Design review of the part built by this model. Coordinates are the model's own, in mm. A direction names the side the tool comes from. Give positions to 0.01 mm unless a question says otherwise; leave off trailing zeros. Order: outer loops, then holes, each group sorted by start corner. A loop starts at its lowest first (then second) coordinate and runs counter-clockwise, first axis right, second up. Notation, with made-up numbers: (28, -10.75) -> (51, -10.75) arc R24 ccw to (51, 27.25) -> close; hole circle Ø3 at (-4.5, -20). An arc over 180 degrees is marked (long way). Return JSON: item names as keys, results as strings.
```python
from build123d import *

# Parameters (mm, degrees)
AUFSATZ_LINEAR_START            = -9.5
AUFSATZ_LINEAR_AUSTRAGEN1_DEPTH = 80


with BuildPart() as part:
    # Skizze1 → Aufsatz-Linear austragen1 (new body)
    with BuildSketch(Plane.XY.offset(AUFSATZ_LINEAR_START)):
        with BuildLine():
            Line((0, 25), (435, 25))
            Line((435, 25), (450, 25))
            ThreePointArc((450, 25), (475, 0), (450, -25))
            Line((450, -25), (0, -25))
            ThreePointArc((0, -25), (-25, 0), (0, 25))
        make_face()
        with BuildLine():
            Line((0, 23), (435, 23))
            Line((435, 23), (450, 23))
            ThreePointArc((450, 23), (473, 0), (450, -23))
            Line((450, -23), (0, -23))
            ThreePointArc((0, -23), (-23, 0), (0, 23))
        make_face(mode=Mode.SUBTRACT)
    extrude(amount=-AUFSATZ_LINEAR_AUSTRAGEN1_DEPTH)


solid = part.part
```
Item 1: Add section A-A (y = 0). Give the boundary of the cut face in (x, z).
Result set:
{"outline": "(-25, -89.5) -> (-23, -89.5) -> (-23, -9.5) -> (-25, -9.5) -> close; (473, -89.5) -> (475, -89.5) -> (475, -9.5) -> (473, -9.5) -> close"}
Item 2: Machinability: for faces 1 (the face through (226, -24, -9.5)), 2 (the face through (-22.994, -0.506, -48.94)), which of the approach directions +Z, -Z, +X, -X, +Y, -Y give a long, thin tool a straight path to every point of the face, cutting with its end or side? Answer none if there is none.
Result set:
{"face 1": "+Z, +X, -X, +Y, -Y", "face 2": "+Z, -Z"}
Item 3: Mouldability with a two-part tool opening along Y and no side actions: class faces 3 (the face through (228, -25, -49)), 4 (the face through (226, -24, -89.5)), 5 (the face through (228, -23, -49)) as released by +Y, released by -Y, zero draft, split by the parting line, or undercut.
Result set:
{"face 3": "released by -Y", "face 4": "zero draft", "face 5": "undercut"}
Item 4: Add section B-B (x = 57.5). Give the boundary of the cut face in (y, z), plus the area to 3 significant figures.
Result set:
{"outline": "(-25, -89.5) -> (-23, -89.5) -> (-23, -9.5) -> (-25, -9.5) -> close; (23, -89.5) -> (25, -89.5) -> (25, -9.5) -> (23, -9.5) -> close", "area": "320 mm^2"}
Item 5: For pin 1 (6 mm diameter, centred on y = 13.5, z = -65, fed in from -X); pin 2 (2 mm diameter, centred on y = 8, z = -29, fed in from -X); pin 3 (10 mm diameter, centred on x = 416, y = -15, fed in from +Z) (3 decimals); pin 4 (4 mm diameter, centred on y = 3, z = -32.5, fed in from -X), all flat-tipped, find the tip position at first contact; note any pin that passes through.
Result set:
{"pin 1": "stops at x = -22.69", "pin 2": "stops at x = -24", "pin 3": "passes through", "pin 4": "stops at x = -24.98"}
Item 6: Wall thickness on L1, parallel to Y at x = 254, z = -33.5; L2, parallel to X at y = -2, z = -24; L3, parallel to X at y = -10.5, z = -39: over which ranges is each line inside the solid? List them lowest first. Write a range as [from, to].
Result set:
{"L1": "y = [-25, -23], [23, 25]", "L2": "x = [-24.92, -22.91], [472.91, 474.92]", "L3": "x = [-22.69, -20.46], [470.46, 472.69]"}
Item 7: Add section C-C (z = -44). Give the boundary of the cut face in (x, y).
Result set:
{"outline": "(0, -25) -> (450, -25) arc R25 ccw to (450, 25) -> (0, 25) arc R25 ccw to start; hole (0, -23) -> (450, -23) arc R23 ccw to (450, 23) -> (0, 23) arc R23 ccw to start"}
